Design review of the part built by this model. Coordinates are the model's own, in mm. A direction names the side the tool comes from. Coordinates: 2 decimals unless noted, no trailing zeros. Loops run counter-clockwise (first coordinate to the right, second up) from the corner with the lowest first, then second, coordinate; pieces in that order, holes last. Notation, with made-up numbers: (-35, 17) -> (24, 17) arc R37 ccw to (24, 53) -> close; hole circle Ø10 at (6.5, 6.5). An arc over 180 degrees is marked (long way). One line per item, written item: value. Start each with the question number.
1. Machinability: for faces 5 (the flat face through (-45, -49, -46)), 6 (the flat face through (-32.76, -21.21, 63.88)), 7 (the flat face through (-30.3, 26, -62)), which of the approach directions +Z, -Z, +X, -X, +Y, -Y give a long, thin tool a straight path to every point of the face, cutting with its end or side? Answer none if there is none.
2. Draft analysis for pull direction Z (two halves, no side actions). For faces 1 (the flat face through (-43, -50.5, -51.2)), 2 (the cylindrical face through (-45.03, 22.9, -72.73)), 3 (the cylindrical face through (-40.082, 0.526, -68.919)), 4 (the flat face through (-45, -1.4, -65.9)), state which applies: pulls with the +Z half, pulls with the -Z half, needs draft (parallel to the pull), parting line crosses it, or undercut.
3. For probe 1 along Y at (x, z) = (-38.5, 0); probe 2 along Y at (x, z) = (-46, -49.5); probe 3 along Y at (x, z) = (-38, 44.5), list the stretches that pass through material, from the lowest coordinate up.
4. Add section B-B on x = -33.5. Write out the cut boundary in (y, z).
5. Add section D-D on z = -28. Write out the cut boundary in (x, y).
6. Insertion check: pin 1 (10 mm diameter, centred on x = -33, y = -26, fed in from -Z); pin 2 (1 mm diameter, centred on x = -37, z = -41, fed in from +Y); pin 3 (7.5 mm diameter, centred on y = 67.25, z = 0, fed in from +X); pin 4 (5 mm diameter, centred on y = -65.5, z = 1, fed in from -X). Each pin has a flat end and moves straight along its axis. Give the tip position at first contact, or say it passes through.
7. Add section A-A on y = 0. Write out the cut boundary in (x, z).
```python
from build123d import *

# Parameters (mm, degrees)
CUT_EXTRUDE_1_DEPTH       = 5
CUT_EXTRUDE_2_DEPTH       = 5
EXTRUDE_1_DEPTH           = 5
HOLE_WIZARD_1_D           = 3.5
HOLE_WIZARD_1_DEPTH       = 16.7
HOLE_WIZARD_1_CBORE_D     = 6.5
HOLE_WIZARD_1_CBORE_DEPTH = 2
HOLE_WIZARD_2_D           = 3.5
HOLE_WIZARD_2_DEPTH       = 16.7
HOLE_WIZARD_2_CBORE_D     = 6.5
HOLE_WIZARD_2_CBORE_DEPTH = 2
HOLE_WIZARD_3_D           = 3.5
HOLE_WIZARD_3_DEPTH       = 16.7
HOLE_WIZARD_3_CBORE_D     = 6.5
HOLE_WIZARD_3_CBORE_DEPTH = 2
HOLE_WIZARD_4_D           = 3.5
HOLE_WIZARD_4_DEPTH       = 16.7
HOLE_WIZARD_4_CBORE_D     = 6.5
HOLE_WIZARD_4_CBORE_DEPTH = 2
HOLE_WIZARD_5_D           = 3.5
HOLE_WIZARD_5_DEPTH       = 16.7
HOLE_WIZARD_5_CBORE_D     = 6.5
HOLE_WIZARD_5_CBORE_DEPTH = 2
HOLE_WIZARD_6_D           = 3.5
HOLE_WIZARD_6_DEPTH       = 16.7
HOLE_WIZARD_6_CBORE_D     = 6.5
HOLE_WIZARD_6_CBORE_DEPTH = 2
HOLE_WIZARD_7_D           = 3.5
HOLE_WIZARD_7_DEPTH       = 16.7
HOLE_WIZARD_7_CBORE_D     = 6.5
HOLE_WIZARD_7_CBORE_DEPTH = 2
HOLE_WIZARD_8_D           = 3.5
HOLE_WIZARD_8_DEPTH       = 16.7
HOLE_WIZARD_8_CBORE_D     = 6.5
HOLE_WIZARD_8_CBORE_DEPTH = 2


with BuildPart() as part:
    # 草图2 → 旋转1 (revolve)
    with BuildSketch(Plane.XY, mode=Mode.PRIVATE) as revolve_1_sk:
        Polygon((-30.3, 71.75), (-43, 71.75), (-43, 76.25), (-47, 76.25), (-47, 62.75), (-30.3, 62.75), align=None)
    revolve(revolve_1_sk.sketch.rotate(Axis((-47, 0, 0), (1, 0, 0)), 270), axis=Axis((-47, 0, 0), (1, 0, 0)))

    # 草图3 → 切除-拉伸1 (cut)
    with BuildSketch(Plane(origin=(-30.3, 0, 0), x_dir=(0, 0, -1), z_dir=(1, 0, 0))):
        with BuildLine():
            Line((55.944003631, 28.422367209), (64.280726218, 31.87555077))
            ThreePointArc((64.280726218, 31.87555077), (-27.457536272, 66.288356458), (-67.992755512, -22.913919305))
            Line((-67.992755512, -22.913919305), (-59.656032925, -19.460735743))
            ThreePointArc((-59.656032925, -19.460735743), (-24.013385381, 57.973440665), (55.944003631, 28.422367209))
        make_face()
    extrude(amount=-CUT_EXTRUDE_1_DEPTH, mode=Mode.SUBTRACT)

    # 草图4 → 切除-拉伸2 (cut)
    with BuildSketch(Plane(origin=(-30.3, 0, 0), x_dir=(0, 0, -1), z_dir=(1, 0, 0))):
        with BuildLine():
            Line((-55.944003631, -28.422367209), (-64.280726218, -31.87555077))
            ThreePointArc((-64.280726218, -31.87555077), (27.457536272, -66.288356458), (67.992755512, 22.913919305))
            Line((67.992755512, 22.913919305), (59.656032925, 19.460735743))
            ThreePointArc((59.656032925, 19.460735743), (24.013385381, -57.973440665), (-55.944003631, -28.422367209))
        make_face()
    extrude(amount=-CUT_EXTRUDE_2_DEPTH, mode=Mode.SUBTRACT)

    # 草图5 → 凸台-拉伸1 (add)
    with BuildSketch(Plane(origin=(-30.3, 0, 0), x_dir=(0, 0, -1), z_dir=(1, 0, 0))):
        with BuildLine():
            Line((55.944003631, 28.422367209), (55.431709583, 28.210168066))
            ThreePointArc((55.431709583, 28.210168066), (56.54956954, 26.875405525), (57.39905958, 25.355679036))
            ThreePointArc((57.39905958, 25.355679036), (56.692271418, 26.898863571), (55.944003631, 28.422367209))
        make_face()
    extrude(amount=-EXTRUDE_1_DEPTH)

    # 孔1
    with Locations(Plane.ZY.offset(47)):
        with Locations((-67.25, 0)):
            CounterBoreHole(HOLE_WIZARD_1_D / 2, HOLE_WIZARD_1_CBORE_D / 2, HOLE_WIZARD_1_CBORE_DEPTH, depth=HOLE_WIZARD_1_DEPTH)

    # 孔2
    with Locations(Plane.ZY.offset(47)):
        with Locations((-47.552931035, 47.552931035)):
            CounterBoreHole(HOLE_WIZARD_2_D / 2, HOLE_WIZARD_2_CBORE_D / 2, HOLE_WIZARD_2_CBORE_DEPTH, depth=HOLE_WIZARD_2_DEPTH)

    # 孔3
    with Locations(Plane.ZY.offset(47)):
        with Locations((0, 67.25)):
            CounterBoreHole(HOLE_WIZARD_3_D / 2, HOLE_WIZARD_3_CBORE_D / 2, HOLE_WIZARD_3_CBORE_DEPTH, depth=HOLE_WIZARD_3_DEPTH)

    # 孔4
    with Locations(Plane.ZY.offset(47)):
        with Locations((47.552931035, 47.552931035)):
            CounterBoreHole(HOLE_WIZARD_4_D / 2, HOLE_WIZARD_4_CBORE_D / 2, HOLE_WIZARD_4_CBORE_DEPTH, depth=HOLE_WIZARD_4_DEPTH)

    # 孔5
    with Locations(Plane.ZY.offset(47)):
        with Locations((67.25, 0)):
            CounterBoreHole(HOLE_WIZARD_5_D / 2, HOLE_WIZARD_5_CBORE_D / 2, HOLE_WIZARD_5_CBORE_DEPTH, depth=HOLE_WIZARD_5_DEPTH)

    # 孔6
    with Locations(Plane.ZY.offset(47)):
        with Locations((47.552931035, -47.552931035)):
            CounterBoreHole(HOLE_WIZARD_6_D / 2, HOLE_WIZARD_6_CBORE_D / 2, HOLE_WIZARD_6_CBORE_DEPTH, depth=HOLE_WIZARD_6_DEPTH)

    # 孔7
    with Locations(Plane.ZY.offset(47)):
        with Locations((0, -67.25)):
            CounterBoreHole(HOLE_WIZARD_7_D / 2, HOLE_WIZARD_7_CBORE_D / 2, HOLE_WIZARD_7_CBORE_DEPTH, depth=HOLE_WIZARD_7_DEPTH)

    # 孔8
    with Locations(Plane.ZY.offset(47)):
        with Locations((-47.552931035, -47.552931035)):
            CounterBoreHole(HOLE_WIZARD_8_D / 2, HOLE_WIZARD_8_CBORE_D / 2, HOLE_WIZARD_8_CBORE_DEPTH, depth=HOLE_WIZARD_8_DEPTH)


solid = part.part
```
Worked answers:
1. face 5: -X
1. face 6: +Z, +X, +Y
1. face 7: +Z, -Z, +X, +Y, -Y
2. face 1: needs draft
2. face 2: parting line crosses it
2. face 3: undercut
2. face 4: undercut
3. probe 1: y = -71.75 to -69, -65.5 to -62.75, 62.75 to 65.5, 69 to 71.75
3. probe 2: y = -58 to -50.16, -44.95 to -38.57, 38.57 to 44.95, 50.16 to 58
3. probe 3: y = -56.28 to -44.24, 44.24 to 56.28
4. outline: (-31.88, 64.28) -> (-28.42, 55.94) arc R62.75 cw to (-19.46, 59.66) -> (-22.91, 67.99) arc R71.75 ccw to start; (19.46, -59.66) -> (22.91, -67.99) arc R71.75 ccw to (31.88, -64.28) -> (28.21, -55.43) arc R9.3 cw to (25.36, -57.4) arc R62.75 cw to start
5. outline: (-47, -70.92) -> (-43, -70.92) -> (-43, -66.06) -> (-35.3, -66.06) -> (-35.3, -56.16) -> (-47, -56.16) -> close; (-47, 56.16) -> (-35.3, 56.16) -> (-35.3, 66.06) -> (-43, 66.06) -> (-43, 70.92) -> (-47, 70.92) -> close
6. pin 1: stops at z = -68.43
6. pin 2: stops at y = 59.23
6. pin 3: stops at x = -35.3
6. pin 4: stops at x = -47
7. outline: (-47, -76.25) -> (-43, -76.25) -> (-43, -71.75) -> (-35.3, -71.75) -> (-35.3, -69) -> (-45, -69) -> (-45, -70.5) -> (-47, -70.5) -> close; (-47, -64) -> (-45, -64) -> (-45, -65.5) -> (-35.3, -65.5) -> (-35.3, -62.75) -> (-47, -62.75) -> close; (-47, 62.75) -> (-35.3, 62.75) -> (-35.3, 65.5) -> (-45, 65.5) -> (-45, 64) -> (-47, 64) -> close; (-47, 70.5) -> (-45, 70.5) -> (-45, 69) -> (-35.3, 69) -> (-35.3, 71.75) -> (-43, 71.75) -> (-43, 76.25) -> (-47, 76.25) -> close
